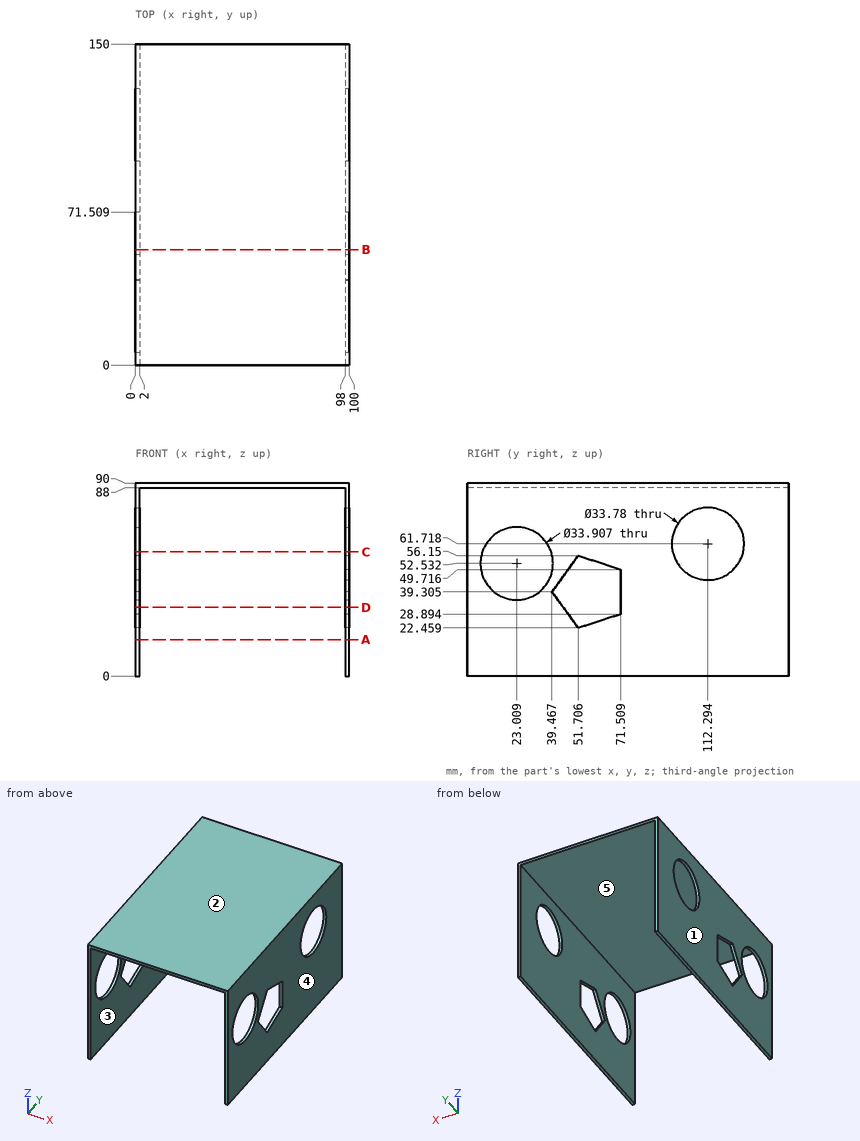
Could you check a few things on this drawing? It's one solid part, dimensions in mm from its lowest x, y, z. A direction names the side the tool comes from. Coordinates: 2 decimals unless noted, no trailing zeros. Order: outer loops, then holes, each group sorted by start corner. A loop starts at its lowest first (then second) coordinate and runs counter-clockwise, first axis right, second up.
1. If we section it at D-D (z = 32): Please give me the cut outline in (x, y) (1 decimal).
2. I need wall thicknesses on line 1 (X direction, y = 38, z = 70); line 2 (Z direction, x = 90.5, y = 45.5). Which ranges of each line are inside material? Lowest first, please.
3. For the marked faces 4 and 5, which set-ups out of +Z, -Z, +X, -X, +Y, -Y let a thin tool reach every point of the face, with its end or its side?
4. If we section it at B-B (y = 54): Please give me the cut outline in (x, z) (1 decimal).
5. If we section it at A-A (z = 17): Please give me the cut outline in (x, y).
6. I'm going to push flat-ended pins straight in: pin 1 (1.5 mm diameter, centred on x = 73, y = 29, fed in from -Z); pin 2 (20.5 mm diameter, centred on y = 112.29, z = 61.72, fed in from +X). Where does each tip first touch, or does it pass through?
7. If we section it at C-C (z = 58): Please give me the cut outline in (x, y).
8. Thinking about a two-plate mould opening in X: for the marked faces 1, 2 and 3, which applies, +X half, -X half, draft (parallel to the pull), parting line (faces both ways), or undercut?
Entries:
1. outline: (0, 0) - (2, 0) - (2, 44.8) - (0, 44.8) - close; (0, 71.5) - (2, 71.5) - (2, 150) - (0, 150) - close; (98, 0) - (100, 0) - (100, 44.8) - (98, 44.8) - close; (98, 71.5) - (100, 71.5) - (100, 150) - (98, 150) - close
2. line 1: x = 0 to 2, 98 to 100
2. line 2: z = 88 to 90
3. face 4: +Z, -Z, +X, +Y, -Y
3. face 5: -Z, +Y, -Y
4. outline: (0, 0) - (2, 0) - (2, 23.2) - (0, 23.2) - close; (0, 55.4) - (2, 55.4) - (2, 88) - (98, 88) - (98, 55.4) - (100, 55.4) - (100, 90) - (0, 90) - close; (98, 0) - (100, 0) - (100, 23.2) - (98, 23.2) - close
5. outline: (0, 0) - (2, 0) - (2, 150) - (0, 150) - close; (98, 0) - (100, 0) - (100, 150) - (98, 150) - close
6. pin 1: stops at z = 88
6. pin 2: passes through
7. outline: (0, 0) - (2, 0) - (2, 6.96) - (0, 6.96) - close; (0, 39.06) - (2, 39.06) - (2, 95.82) - (0, 95.82) - close; (0, 128.77) - (2, 128.77) - (2, 150) - (0, 150) - close; (98, 0) - (100, 0) - (100, 6.96) - (98, 6.96) - close; (98, 39.06) - (100, 39.06) - (100, 95.82) - (98, 95.82) - close; (98, 128.77) - (100, 128.77) - (100, 150) - (98, 150) - close
8. face 1: -X half
8. face 2: draft
8. face 3: undercut
